Build history of the part. All positions in model axes, mm. Face numbers are marked on the shaded views. A direction names the side the tool comes from. Coordinates: 2 decimals unless noted, no trailing zeros. Order: outer loops, then holes, each group sorted by start corner. A loop starts at its lowest first (then second) coordinate and runs counter-clockwise, first axis right, second up. Notation, with made-up numbers: M 19.5,43.25 L 33.5,43.25 A28 cw 33.5,71.25 Z; hole C -0.5,-9.75 d3. An arc over 180 degrees is marked long. Write item = value, one per line. Start each with the question number.
Q1. Pin check, flat tips, straight feed: P1, Ø1.5, axis at y = -34.5, z = 9.5, coming from the -X side; P2, Ø1, axis at y = -29, z = 11.5, coming from the -X side; P3, Ø8, axis at x = -11.89, y = -2.79, coming from the -Z side; P4, Ø1.5, axis at x = 15.5, z = 20, coming from the -Y side. Stop position of each tip, or through.
Q2. 3-axis set-ups, long thin cutter, end or side, ignore diameter. For the marked faces 1, 2 and 3: which of +Z, -Z, +X, -X, +Y, -Y reach the whole face in a straight line?
Q3. Drill centre lines: probe 1 along X at (y, z) = (-2.5, 13.5); probe 2 along Y at (x, z) = (47, 23); probe 3 along Y at (x, z) = (-11, 4.5). Where is each one in solid material? Low to high.
Q4. Band-saw the part on A-A on z = 24.5. Write the cut outline in (x, y).
Q5. Band-saw the part on B-B on x = 69. Write the cut outline in (y, z).
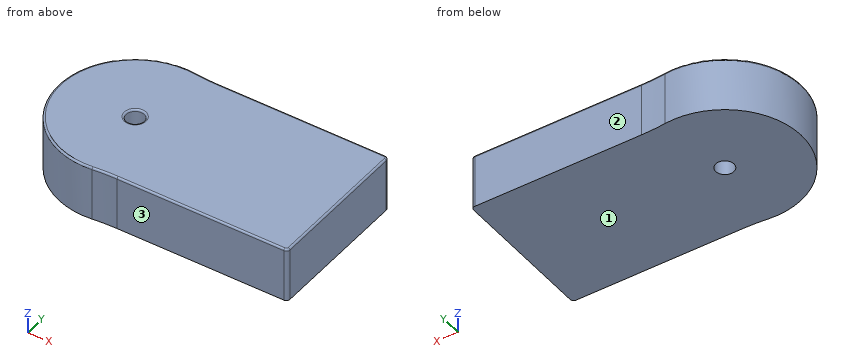
```python
from build123d import *

# Parameters (mm, degrees)
SKETCH_1_R      = 5
EXTRUDE_1_DEPTH = 30
FILLET_1_R      = 120
FILLET_2_R      = 1
FILLET_3_R      = 1
FILLET_4_R      = 2


with BuildPart() as part:
    # 草图1 → 凸台-拉伸1 (new body)
    with BuildSketch(Plane.XY):
        with BuildLine():
            Line((-2.776926107, -43.794806673), (99.984598045, -43.794806673))
            Line((99.984598045, -43.794806673), (99.984598045, 38.205193327))
            Line((99.984598045, 38.205193327), (-2.776926107, 38.205193327))
            ThreePointArc((-2.776926107, 38.205193327), (-53.887359686, -2.794806673), (-2.776926107, -43.794806673))
        make_face()
        with Locations((-11.887359686, -2.794806673)):
            Circle(SKETCH_1_R, mode=Mode.SUBTRACT)
    extrude(amount=EXTRUDE_1_DEPTH)

    # 圆角1
    fillet_1_edges = [part.edges().sort_by_distance(p)[0] for p in [
        (-2.776926107, 38.205193327, 15),
        (-2.776926107, -43.794806673, 15),
    ]]
    fillet(fillet_1_edges, radius=FILLET_1_R)

    # 圆角2
    fillet_2_edges = [part.edges().sort_by_distance(p)[0] for p in [
        (-16.887359686, -2.794806673, 30),
    ]]
    fillet(fillet_2_edges, radius=FILLET_2_R)

    # 圆角3
    fillet_3_edges = [part.edges().sort_by_distance(p)[0] for p in [
        (99.984598045, -2.794806673, 30),
        (-53.887359686, -2.794806673, 30),
        (53.034719557, 38.205193327, 30),
        (53.034719557, -43.794806673, 30),
        (-0.581825597, 38.390521623, 30),
        (-0.581825597, -43.980134969, 30),
    ]]
    fillet(fillet_3_edges, radius=FILLET_3_R)

    # 圆角4
    # the kernel refuses this fillet: 2 mm, written as the material it takes off along each edge
    with BuildSketch(Plane(origin=(97.984598045, -41.794806673, 30), x_dir=(0, -1, 0), z_dir=(-1, 0, 0))) as fillet_4_piece_1:
        with BuildLine():
            CenterArc((1, -1), 1, 0, 90)
            Line((2, -1), (2, 0))
            Line((2, 0), (1, 0))
        make_face()
    revolve(axis=Axis((97.984598045, -41.794806673, 30), (0, 0, 1)), revolution_arc=90, mode=Mode.SUBTRACT)
    with BuildSketch(Plane(origin=(97.984598045, 36.205193327, 30), x_dir=(1, 0, 0), z_dir=(0, -1, 0))) as fillet_4_piece_2:
        with BuildLine():
            CenterArc((1, -1), 1, 0, 90)
            Line((2, -1), (2, 0))
            Line((2, 0), (1, 0))
        make_face()
    revolve(axis=Axis((97.984598045, 36.205193327, 30), (0, 0, 1)), revolution_arc=90, mode=Mode.SUBTRACT)
    with BuildSketch(Plane(origin=(99.984598045, 38.205193327, -5), x_dir=(0, -1, 0), z_dir=(0, 0, 1))) as fillet_4_piece_3:
        with BuildLine():
            CenterArc((FILLET_4_R, -FILLET_4_R), FILLET_4_R, 90, 90)
            Line((0, -FILLET_4_R), (0, 0))
            Line((0, 0), (FILLET_4_R, 0))
        make_face()
    extrude(amount=35, mode=Mode.SUBTRACT)
    with BuildSketch(Plane(origin=(99.984598045, -43.794806673, -5), x_dir=(0, 1, 0), z_dir=(0, 0, 1))) as fillet_4_piece_4:
        with BuildLine():
            CenterArc((FILLET_4_R, FILLET_4_R), FILLET_4_R, 180, 90)
            Line((0, FILLET_4_R), (0, 0))
            Line((0, 0), (FILLET_4_R, 0))
        make_face()
    extrude(amount=35, mode=Mode.SUBTRACT)


solid = part.part
```
Recorded:
q1.P1 = -40.27
q1.P2 = -45.1
q1.P3 = through
q1.P4 = -43.79
q2.face_1 = -Z, +X, -X, +Y, -Y
q2.face_2 = +Z, -Z, +X, +Y
q2.face_3 = +Z, -Z, +X, -Y
q3.probe_1 = -53.89 to -16.88, -6.9 to 99.98
q3.probe_2 = -43.79 to 38.21
q3.probe_3 = -44.79 to -7.72, 2.13 to 39.2
q4.outline = M -7.23,-44.54 A120 cw 6.08,-43.79 L 97.98,-43.79 A2 ccw 99.98,-41.79 L 99.98,36.21 A2 ccw 97.98,38.21 L 6.08,38.21 A120 cw -7.23,38.95 A42 ccw long Z; hole C -11.89,-2.79 d10
q5.outline = M -43.79,0 L 38.21,0 L 38.21,29 A1 ccw 37.21,30 L -42.79,30 A1 ccw -43.79,29 Z
